```python
from build123d import *

# Parameters (mm, degrees)
BOSS_EXTRUDE1_DEPTH = 20
FILLET1_R           = 10
CUT_EXTRUDE1_DEPTH  = 52.983170353
SKETCH3_R           = 2.1
CUT_EXTRUDE2_DEPTH  = 52.983170353
SKETCH4_R           = 2.6
CUT_EXTRUDE3_DEPTH  = 52.983170353


with BuildPart() as part:
    # Sketch1 → Boss-Extrude1 (new body)
    with BuildSketch(Plane(origin=(0, 0, 0), x_dir=(1, 0, 0), z_dir=(0, 1, 0))):
        with BuildLine():
            Line((0, 0), (40, 0))
            Line((40, 0), (40, -6))
            Line((40, -6), (13.955285737, -6))
            ThreePointArc((13.955285737, -6), (0, -26.5), (-13.955285737, -6))
            Line((-13.955285737, -6), (-40, -6))
            Line((-40, -6), (-40, 0))
            Line((-40, 0), (0, 0))
        make_face()
    extrude(amount=BOSS_EXTRUDE1_DEPTH)

    # Fillet1
    fillet1_edges = [part.edges().sort_by_distance(p)[0] for p in [
        (13.955285737, 10, 6),
        (-13.955285737, 10, 6),
    ]]
    fillet(fillet1_edges, radius=FILLET1_R)

    # Sketch2 → Cut-Extrude1 (cut, through all)
    with BuildSketch(Plane(origin=(0, 20, 0), x_dir=(1, 0, 0), z_dir=(0, 1, 0))):
        Polygon((-7.043673284, -11.5), (-3.521836642, -17.6), (3.521836642, -17.6), (7.043673284, -11.5), (3.521836642, -5.4), (-3.521836642, -5.4), align=None)
    extrude(amount=-CUT_EXTRUDE1_DEPTH, mode=Mode.SUBTRACT)

    # Sketch3 → Cut-Extrude2 (cut, through all)
    with BuildSketch(Plane(origin=(0, 20, 0), x_dir=(1, 0, 0), z_dir=(0, 1, 0))):
        with Locations(Location((0, -21.5, 0), (0, 0, 270))):
            Circle(SKETCH3_R)
    extrude(amount=-CUT_EXTRUDE2_DEPTH, mode=Mode.SUBTRACT)

    # Sketch4 → Cut-Extrude3 (cut, through all)
    with BuildSketch(Plane(origin=(0, 0, 0), x_dir=(-1, 0, 0), z_dir=(0, 0, -1))):
        with Locations((-30, 10)):
            Circle(SKETCH4_R)
        with Locations((30, 10)):
            Circle(SKETCH4_R)
    extrude(amount=-CUT_EXTRUDE3_DEPTH, mode=Mode.SUBTRACT)


solid = part.part
```
Could you check a few things on this model? Use its own coordinates, in mm. A direction names the side the tool comes from. Coordinates: 2 decimals unless noted, no trailing zeros. Write each loop counter-clockwise with the first axis right and the second up, starting at its lowest first coordinate (ties: lowest second). Pieces come first, ordered by that corner, then holes. Notation, with made-up numbers: (-39, -7) - (-15, -7) arc R20 ccw to (-15, -1) - close; hole circle Ø1 at (30.5, -37.75). An arc over 180 degrees is marked (long way). Use a Markdown table: item, result.
Q1. Imagine slicing it at B-B (x = -30). List the corners of the cut face in (y, z) for me, and give its area (3 significant figures).
Geometry check:
| item | result |
|---|---|
| outline | (0, 0) - (7.4, 0) - (7.4, 6) - (0, 6) - close; (12.6, 0) - (20, 0) - (20, 6) - (12.6, 6) - close |
| area | 88.8 mm2 |
Q2. Thinking about a two-plate mould opening in Z: for faces 5 (the cylindrical face through (18.26, 10.14, 8.26)), 6 (the flat face through (40, 10, 3)), 7 (the flat face through (5.26, 10.14, 14.59)), which applies, +Z half, -Z half, draft (parallel to the pull), parting line (faces both ways), or undercut?
Geometry check:
| item | result |
|---|---|
| face 5 | +Z half |
| face 6 | draft |
| face 7 | undercut |
Q3. Please list where these lines run through material, in increasing order: L1, parallel to Y at x = -30, z = 2.2; L2, parallel to X at y = 7.5, z = 11.25; L3, parallel to Z at x = -5.5, y = 17.75.
Geometry check:
| item | result |
|---|---|
| L1 | y = 0 to 7.4, 12.6 to 20 |
| L2 | x = -15.79 to -6.9, 6.9 to 15.79 |
| L3 | z = 0 to 8.83, 14.17 to 25.46 |
Q4. Which directions (+Z, -Z, +X, -X, +Y, -Y) give clear straight access to the entire face, cutting with the end or side of a thin tool? Please do faces 1 (the flat face through (34, 10, 6)), 2 (the flat face through (-1, 10, 0)), 3 (the flat face through (-34, 10, 6)), 4 (the flat face through (0, 10, 17.6)).
Geometry check:
| item | result |
|---|---|
| face 1 | +Z, +X, +Y, -Y |
| face 2 | -Z, +X, -X, +Y, -Y |
| face 3 | +Z, -X, +Y, -Y |
| face 4 | +Y, -Y |
Q5. Imagine slicing it at C-C (z = 7.5). List the corners of the cut face in (x, y) for me, and give its area (3 significant figures).
Geometry check:
| item | result |
|---|---|
| outline | (-19.32, 0) - (-4.73, 0) - (-4.73, 20) - (-19.32, 20) - close; (4.73, 0) - (19.32, 0) - (19.32, 20) - (4.73, 20) - close |
| area | 584 mm2 |
Q6. Imagine slicing it at A-A (y = 10). List the corners of the cut face in (x, z) for me (3 decimals), and give its area (3 significant figures).
Geometry check:
| item | result |
|---|---|
| outline | (-40, 0) - (-32.6, 0) - (-32.6, 6) - (-40, 6) - close; (-27.4, 0) - (27.4, 0) - (27.4, 6) - (24.592, 6) arc R10 cw to (14.755, 14.2) arc R15 ccw to (-14.755, 14.2) arc R10 cw to (-24.592, 6) - (-27.4, 6) - close; (32.6, 0) - (40, 0) - (40, 6) - (32.6, 6) - close; hole (-7.044, 11.5) - (-3.522, 5.4) - (3.522, 5.4) - (7.044, 11.5) - (3.522, 17.6) - (-3.522, 17.6) - close; hole circle Ø4.2 at (0, 21.5) |
| area | 830 mm2 |
Q7. Imagine slicing it at D-D (z = 2). List the corners of the cut face in (x, y) for me.
Geometry check:
| item | result |
|---|---|
| outline | (-40, 0) - (40, 0) - (40, 20) - (-40, 20) - close; hole circle Ø5.2 at (-30, 10); hole circle Ø5.2 at (30, 10) |
Q8. I'm going to push flat-ended pins straight in: pin 1 Ø3 at (x, y) = (12, 12.5) entering from +Z; pin 2 Ø5 at (x, y) = (-12.5, 2.5) entering from -Z; pin 3 Ø3 at (x, y) = (21, 11) entering from +Z; pin 4 Ø4 at (y, z) = (10, 11) entering from -X. Where does each tip first touch, or does it pass through?
Geometry check:
| item | result |
|---|---|
| pin 1 | stops at z = 22.21 |
| pin 2 | stops at z = 0 |
| pin 3 | stops at z = 7.39 |
| pin 4 | stops at x = -17.45 |
